The model under review builds one solid part; all positions refer to its coordinate system, in mm. Coordinates: 2 decimals unless noted, no trailing zeros. Loops run counter-clockwise (first coordinate to the right, second up) from the corner with the lowest first, then second, coordinate; pieces in that order, holes last. Notation, with made-up numbers: (6.25, -2) - (36.25, -2) arc R18 ccw to (36.25, 11) - close; hole circle Ø2 at (10, 58.25). An arc over 180 degrees is marked (long way). Use a Markdown table: item, result. Add a question column.
1) Add section A-A, the plane z = 6. Give the boundary of the cut face in (x, y), and give its area (3 significant figures).
2) Add section B-B, the plane y = 4.6. Give the boundary of the cut face in (x, z).
3) Add section D-D, the plane z = -9. Give the boundary of the cut face in (x, y).
4) Clearance check with flat-ended pins moving along their axes: pin 1 (2 mm diameter, centred on x = 9, y = 2.5, fed in from -Z); pin 2 (1.5 mm diameter, centred on x = 9.5, y = 2.5, fed in from -Z); pin 3 (2 mm diameter, centred on x = -6, z = -6, fed in from +Y). State where each tip first meets the part, or that it passes through.
5) Add section C-C, the plane x = 5.25. Give the boundary of the cut face in (y, z), and give its area (3 significant figures).
6) To check wall thickness, follow L1, parallel to Y at x = 9.5, z = 9.25; L2, parallel to X at y = 1.95, z = -9.5; L3, parallel to Z at x = -6.5, y = 0.5. State the ranges of each line that lie inside material, in increasing order. Write a range as [from, to].
```python
from build123d import *

# Parameters (mm, degrees)
SKETCH1_W           = 26
SKETCH1_H           = 26
SKETCH1_R           = 1.25
BOSS_EXTRUDE1_DEPTH = 5
SKETCH2_R           = 1.25
CUT_EXTRUDE1_DEPTH  = 10
LPATTERN1_COUNT     = 2
LPATTERN1_PITCH     = 16


with BuildPart() as part:
    # Sketch1 → Boss-Extrude1 (new body)
    with BuildSketch(Plane(origin=(0, 0, 0), x_dir=(1, 0, 0), z_dir=(0, 1, 0))):
        Rectangle(SKETCH1_W, SKETCH1_H)
        with Locations(Location((-6, -6, 0), (0, 0, 270))):
            Circle(SKETCH1_R, mode=Mode.SUBTRACT)
        with Locations(Location((6, -6, 0), (0, 0, 270))):
            Circle(SKETCH1_R, mode=Mode.SUBTRACT)
        with Locations(Location((6, 6, 0), (0, 0, 270))):
            Circle(SKETCH1_R, mode=Mode.SUBTRACT)
        with Locations(Location((-6, 6, 0), (0, 0, 270))):
            Circle(SKETCH1_R, mode=Mode.SUBTRACT)
    extrude(amount=BOSS_EXTRUDE1_DEPTH)

    # Sketch2 → Cut-Extrude1 (cut)
    with BuildSketch(Plane.XY.offset(13)):
        with Locations((-9.5, 2.5)):
            Circle(SKETCH2_R)
        with Locations(Location((9.5, 2.5, 0), (0, 0, 180))):
            Circle(SKETCH2_R)
    cut_extrude1 = extrude(amount=-CUT_EXTRUDE1_DEPTH, mode=Mode.SUBTRACT)

    # LPattern1: Cut-Extrude1 ×2
    with Locations(*[(0, 0, -i * LPATTERN1_PITCH) for i in range(1, LPATTERN1_COUNT)]):
        add(cut_extrude1, mode=Mode.SUBTRACT)


solid = part.part
```
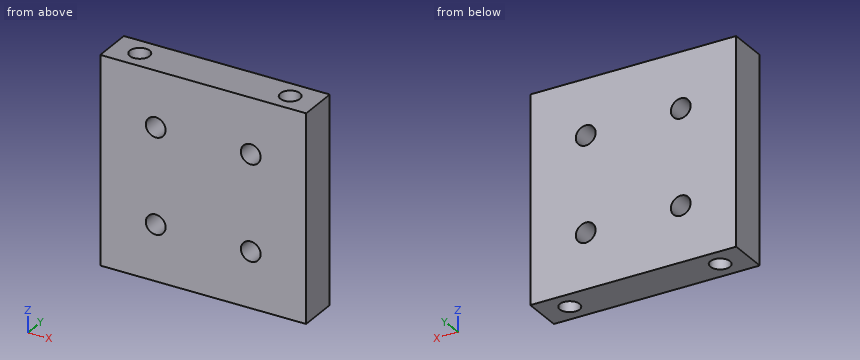
From the geometry:
| question | item | result |
|---|---|---|
| 1 | outline | (-13, 0) - (-7.25, 0) - (-7.25, 5) - (-13, 5) - close; (-4.75, 0) - (4.75, 0) - (4.75, 5) - (-4.75, 5) - close; (7.25, 0) - (13, 0) - (13, 5) - (7.25, 5) - close; hole circle Ø2.5 at (-9.5, 2.5); hole circle Ø2.5 at (9.5, 2.5) |
| 1 | area | 95.2 mm^2 |
| 2 | outline | (-13, -13) - (13, -13) - (13, 13) - (-13, 13) - close; hole circle Ø2.5 at (-6, -6); hole circle Ø2.5 at (-6, 6); hole circle Ø2.5 at (6, -6); hole circle Ø2.5 at (6, 6) |
| 3 | outline | (-13, 0) - (13, 0) - (13, 5) - (-13, 5) - close; hole circle Ø2.5 at (-9.5, 2.5); hole circle Ø2.5 at (9.5, 2.5) |
| 4 | pin 1 | stops at z = -13 |
| 4 | pin 2 | stops at z = -3 |
| 4 | pin 3 | passes through |
| 5 | outline | (0, -13) - (5, -13) - (5, -7) - (0, -7) - close; (0, -5) - (5, -5) - (5, 5) - (0, 5) - close; (0, 7) - (5, 7) - (5, 13) - (0, 13) - close |
| 5 | area | 110 mm^2 |
| 6 | L1 | y = [0, 1.25], [3.75, 5] |
| 6 | L2 | x = [-13, -10.62], [-8.38, 8.38], [10.62, 13] |
| 6 | L3 | z = [-13, -7.15], [-4.85, 4.85], [7.15, 13] |
